The listing builds one solid part. Answer for the finished solid, in the listing's coordinates (mm). Give positions to 0.01 mm unless a question says otherwise; leave off trailing zeros. Order: outer loops, then holes, each group sorted by start corner. A loop starts at its lowest first (then second) coordinate and runs counter-clockwise, first axis right, second up. Notation, with made-up numbers: (30, 78) - (77, 78) arc R12 cw to (77, 92) - close; hole circle Ø2 at (-21.75, -14). An arc over 180 degrees is marked (long way). Answer as a JSON object with one key per item and string values. Group by question number.
Q1. A cutting plane is placed at B-B, the plane y = -8. Give the vertices of the cut face in (x, z), and give its area (3 significant figures).
Q2. Given pin 1 (3 mm diameter, centred on y = -56, z = -3.5, fed in from -X); pin 2 (3 mm diameter, centred on x = 51.5, z = -3, fed in from +Y); pin 3 (2 mm diameter, centred on y = 142.5, z = -4, fed in from +X), each flat-ended and moving along its own axis, determine where each tip first touches the part or whether it passes through.
Q3. A cutting plane is placed at C-C, the plane z = -2.55. Count the separate pieces of the cut face and the enclosed holes in it, and give its area (3 significant figures).
Q4. A cutting plane is placed at D-D, the plane y = 165. Give the vertices of the cut face in (x, z).
Q5. Consider line 1 (Y direction, x = 4, z = -3.7); line 2 (X direction, y = -11, z = -0.4); line 3 (X direction, y = -57, z = -2.95). Determine where each line is inside the solid, lowest interval first.
Q6. A cutting plane is placed at A-A, the plane y = 114.5. Give the vertices of the cut face in (x, z), and give its area (3 significant figures).
from build123d import *

# Parameters (mm, degrees)
SCHIZZO1_R                   = 1.25
ESTRUSIONE_ESTRUSIONE1_DEPTH = 6


with BuildPart() as part:
    # Schizzo1 → Estrusione-Estrusione1 (new body)
    with BuildSketch(Plane.XY):
        Polygon((-110.280237788, 184.011080088), (-104.511080088, 189.780237788), (-98.133615912, 188.947324411), (-82.653889721, 173.46759822), (82.653889721, 173.46759822), (98.133615912, 188.947324411), (104.511080088, 189.780237788), (110.280237788, 184.011080088), (109.447324411, 177.633615912), (83.818771539, 152.00506304), (83.818771539, 86.400644995), (102.629005707, 67.590410826), (102.629005707, 42.409589174), (83.818771539, 23.599355005), (83.818771539, -23.599355005), (102.629005707, -42.409589174), (102.629005707, -67.590410826), (83.818771539, -86.400644995), (83.818771539, -152.00506304), (109.447324411, -177.633615912), (110.280237788, -184.011080088), (104.511080088, -189.780237788), (98.133615912, -188.947324411), (82.653889721, -173.46759822), (-82.653889721, -173.46759822), (-98.133615912, -188.947324411), (-104.511080088, -189.780237788), (-110.280237788, -184.011080088), (-109.447324411, -177.633615912), (-83.818771539, -152.00506304), (-83.818771539, -86.400644995), (-102.629005707, -67.590410826), (-102.629005707, -42.409589174), (-83.818771539, -23.599355005), (-83.818771539, 23.599355005), (-102.629005707, 42.409589174), (-102.629005707, 67.590410826), (-83.818771539, 86.400644995), (-83.818771539, 152.00506304), (-109.447324411, 177.633615912), align=None)
        with Locations((-95, 55)):
            Circle(SCHIZZO1_R, mode=Mode.SUBTRACT)
        with Locations((-75, 55)):
            Circle(SCHIZZO1_R, mode=Mode.SUBTRACT)
        with Locations((-104.5, 184)):
            Circle(SCHIZZO1_R, mode=Mode.SUBTRACT)
        with Locations((0, 20.5)):
            Circle(SCHIZZO1_R, mode=Mode.SUBTRACT)
        with Locations((104.5, 184)):
            Circle(SCHIZZO1_R, mode=Mode.SUBTRACT)
        with Locations((75, 55)):
            Circle(SCHIZZO1_R, mode=Mode.SUBTRACT)
        with Locations((95, 55)):
            Circle(SCHIZZO1_R, mode=Mode.SUBTRACT)
        with Locations((95, -55)):
            Circle(SCHIZZO1_R, mode=Mode.SUBTRACT)
        with Locations((75, -55)):
            Circle(SCHIZZO1_R, mode=Mode.SUBTRACT)
        with Locations((104.5, -184)):
            Circle(SCHIZZO1_R, mode=Mode.SUBTRACT)
        with Locations((0, -20.5)):
            Circle(SCHIZZO1_R, mode=Mode.SUBTRACT)
        with Locations((-104.5, -184)):
            Circle(SCHIZZO1_R, mode=Mode.SUBTRACT)
        with Locations((-75, -55)):
            Circle(SCHIZZO1_R, mode=Mode.SUBTRACT)
        with Locations((-95, -55)):
            Circle(SCHIZZO1_R, mode=Mode.SUBTRACT)
        with BuildLine():
            Line((-59.232107436, 63.271672811), (-59.232107436, -63.271672811))
            ThreePointArc((-59.232107436, -63.271672811), (-59.085980675, -64.022108692), (-58.668953425, -64.662885808))
            Line((-58.668953425, -64.662885808), (-55.942526616, -67.478741779))
            ThreePointArc((-55.942526616, -67.478741779), (-55.285928666, -67.929053421), (-54.505680627, -68.087528781))
            Line((-54.505680627, -68.087528781), (-44.774099334, -68.087528781))
            ThreePointArc((-44.774099334, -68.087528781), (-44.179960459, -67.997240539), (-43.639465339, -67.734527779))
            Line((-43.639465339, -67.734527779), (-12.106917048, -46.011441546))
            ThreePointArc((-12.106917048, -46.011441546), (-11.471061282, -45.294693055), (-11.241551043, -44.364442549))
            Line((-11.241551043, -44.364442549), (-11.241551043, 44.364442549))
            ThreePointArc((-11.241551043, 44.364442549), (-11.471061282, 45.294693055), (-12.106917048, 46.011441546))
            Line((-12.106917048, 46.011441546), (-43.639465339, 67.734527779))
            ThreePointArc((-43.639465339, 67.734527779), (-44.179960459, 67.997240539), (-44.774099334, 68.087528781))
            Line((-44.774099334, 68.087528781), (-54.505680627, 68.087528781))
            ThreePointArc((-54.505680627, 68.087528781), (-55.285928666, 67.929053421), (-55.942526616, 67.478741779))
            Line((-55.942526616, 67.478741779), (-58.668953425, 64.662885808))
            ThreePointArc((-58.668953425, 64.662885808), (-59.085980675, 64.022108692), (-59.232107436, 63.271672811))
        make_face(mode=Mode.SUBTRACT)
        with BuildLine():
            Line((79, 45), (79, 65))
            ThreePointArc((79, 65), (85, 71), (91, 65))
            Line((91, 65), (91, 45))
            ThreePointArc((91, 45), (85, 39), (79, 45))
        make_face(mode=Mode.SUBTRACT)
        with BuildLine():
            Line((-47.48302182, 123.938863738), (-47.48302182, 97.979582184))
            ThreePointArc((-47.48302182, 97.979582184), (-47.253511581, 97.049331677), (-46.617655815, 96.332583186))
            Line((-46.617655815, 96.332583186), (-10.046187512, 71.138134825))
            ThreePointArc((-10.046187512, 71.138134825), (-9.505692391, 70.875422065), (-8.911553517, 70.785133823))
            Line((-8.911553517, 70.785133823), (8.911553517, 70.785133823))
            ThreePointArc((8.911553517, 70.785133823), (9.505692391, 70.875422065), (10.046187512, 71.138134825))
            Line((10.046187512, 71.138134825), (46.617655815, 96.332583186))
            ThreePointArc((46.617655815, 96.332583186), (47.253511581, 97.049331677), (47.48302182, 97.979582184))
            Line((47.48302182, 97.979582184), (47.48302182, 123.938863738))
            ThreePointArc((47.48302182, 123.938863738), (47.330780885, 124.704230603), (46.897235382, 125.353077301))
            Line((46.897235382, 125.353077301), (38.068808258, 134.181504425))
            ThreePointArc((38.068808258, 134.181504425), (37.41996156, 134.615049928), (36.654594695, 134.767290863))
            Line((36.654594695, 134.767290863), (-36.654594695, 134.767290863))
            ThreePointArc((-36.654594695, 134.767290863), (-37.41996156, 134.615049928), (-38.068808258, 134.181504425))
            Line((-38.068808258, 134.181504425), (-46.897235382, 125.353077301))
            ThreePointArc((-46.897235382, 125.353077301), (-47.330780885, 124.704230603), (-47.48302182, 123.938863738))
        make_face(mode=Mode.SUBTRACT)
        with BuildLine():
            Line((-79, 45), (-79, 65))
            ThreePointArc((-79, 65), (-85, 71), (-91, 65))
            Line((-91, 65), (-91, 45))
            ThreePointArc((-91, 45), (-85, 39), (-79, 45))
        make_face(mode=Mode.SUBTRACT)
        with BuildLine():
            Line((91, -45), (91, -65))
            ThreePointArc((91, -65), (85, -71), (79, -65))
            Line((79, -65), (79, -45))
            ThreePointArc((79, -45), (85, -39), (91, -45))
        make_face(mode=Mode.SUBTRACT)
        with BuildLine():
            Line((-79, -45), (-79, -65))
            ThreePointArc((-79, -65), (-85, -71), (-91, -65))
            Line((-91, -65), (-91, -45))
            ThreePointArc((-91, -45), (-85, -39), (-79, -45))
        make_face(mode=Mode.SUBTRACT)
        with BuildLine():
            Line((43.639465339, 67.734527779), (12.106917048, 46.011441546))
            ThreePointArc((12.106917048, 46.011441546), (11.471061282, 45.294693055), (11.241551043, 44.364442549))
            Line((11.241551043, 44.364442549), (11.241551043, -44.364442549))
            ThreePointArc((11.241551043, -44.364442549), (11.471061282, -45.294693055), (12.106917048, -46.011441546))
            Line((12.106917048, -46.011441546), (43.639465339, -67.734527779))
            ThreePointArc((43.639465339, -67.734527779), (44.179960459, -67.997240539), (44.774099334, -68.087528781))
            Line((44.774099334, -68.087528781), (54.505680627, -68.087528781))
            ThreePointArc((54.505680627, -68.087528781), (55.285928666, -67.929053421), (55.942526616, -67.478741779))
            Line((55.942526616, -67.478741779), (58.668953425, -64.662885808))
            ThreePointArc((58.668953425, -64.662885808), (59.085980675, -64.022108692), (59.232107436, -63.271672811))
            Line((59.232107436, -63.271672811), (59.232107436, 63.271672811))
            ThreePointArc((59.232107436, 63.271672811), (59.085980675, 64.022108692), (58.668953425, 64.662885808))
            Line((58.668953425, 64.662885808), (55.942526616, 67.478741779))
            ThreePointArc((55.942526616, 67.478741779), (55.285928666, 67.929053421), (54.505680627, 68.087528781))
            Line((54.505680627, 68.087528781), (44.774099334, 68.087528781))
            ThreePointArc((44.774099334, 68.087528781), (44.179960459, 67.997240539), (43.639465339, 67.734527779))
        make_face(mode=Mode.SUBTRACT)
        with BuildLine():
            Line((-36.654594695, -134.767290863), (36.654594695, -134.767290863))
            ThreePointArc((36.654594695, -134.767290863), (37.41996156, -134.615049928), (38.068808258, -134.181504425))
            Line((38.068808258, -134.181504425), (46.897235382, -125.353077301))
            ThreePointArc((46.897235382, -125.353077301), (47.330780885, -124.704230603), (47.48302182, -123.938863738))
            Line((47.48302182, -123.938863738), (47.48302182, -97.979582184))
            ThreePointArc((47.48302182, -97.979582184), (47.253511581, -97.049331677), (46.617655815, -96.332583186))
            Line((46.617655815, -96.332583186), (10.046187512, -71.138134825))
            ThreePointArc((10.046187512, -71.138134825), (9.505692391, -70.875422065), (8.911553517, -70.785133823))
            Line((8.911553517, -70.785133823), (-8.911553517, -70.785133823))
            ThreePointArc((-8.911553517, -70.785133823), (-9.505692391, -70.875422065), (-10.046187512, -71.138134825))
            Line((-10.046187512, -71.138134825), (-46.617655815, -96.332583186))
            ThreePointArc((-46.617655815, -96.332583186), (-47.253511581, -97.049331677), (-47.48302182, -97.979582184))
            Line((-47.48302182, -97.979582184), (-47.48302182, -123.938863738))
            ThreePointArc((-47.48302182, -123.938863738), (-47.330780885, -124.704230603), (-46.897235382, -125.353077301))
            Line((-46.897235382, -125.353077301), (-38.068808258, -134.181504425))
            ThreePointArc((-38.068808258, -134.181504425), (-37.41996156, -134.615049928), (-36.654594695, -134.767290863))
        make_face(mode=Mode.SUBTRACT)
    extrude(amount=-ESTRUSIONE_ESTRUSIONE1_DEPTH)


solid = part.part
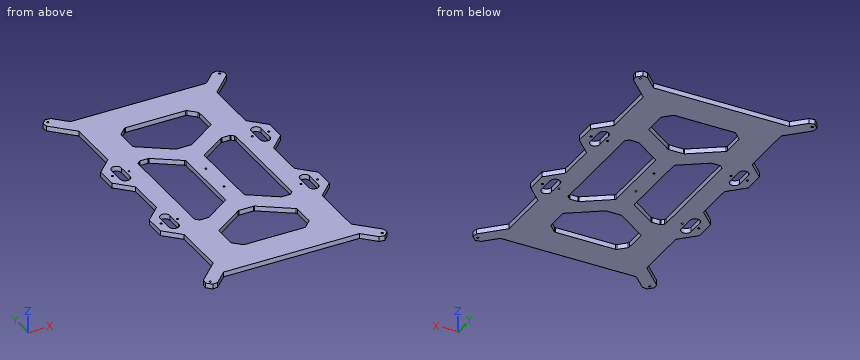
Reply:
{
 "1": {"outline": "(-83.82, -6) - (-59.23, -6) - (-59.23, 0) - (-83.82, 0) - close; (-11.24, -6) - (11.24, -6) - (11.24, 0) - (-11.24, 0) - close; (59.23, -6) - (83.82, -6) - (83.82, 0) - (59.23, 0) - close", "area": "430 mm^2"},
 "2": {"pin 1": "stops at x = -102.63", "pin 2": "stops at y = 173.47", "pin 3": "stops at x = 83.82"},
 "3": {"separate pieces": "1", "enclosed holes": "22", "area": "40,500 mm^2"},
 "4": {"outline": "(-96.81, -6) - (96.81, -6) - (96.81, 0) - (-96.81, 0) - close"},
 "5": {"line 1": "y = -173.47 to -134.77, -70.79 to 70.79, 134.77 to 173.47", "line 2": "x = -83.82 to -59.23, -11.24 to 11.24, 59.23 to 83.82", "line 3": "x = -102.63 to -91, -79 to -59.23, -28.06 to 28.06, 59.23 to 79, 91 to 102.63"},
 "6": {"outline": "(-83.82, -6) - (-47.48, -6) - (-47.48, 0) - (-83.82, 0) - close; (47.48, -6) - (83.82, -6) - (83.82, 0) - (47.48, 0) - close", "area": "436 mm^2"}
}
